Can you work these out from the model? Positions are in its coordinate system, mm. Round coordinates to 2 decimals unless told otherwise and drop trailing zeros. Loops run counter-clockwise (first coordinate to the right, second up) from the corner with the lowest first, then second, coordinate; pieces in that order, holes last. Notation, with made-up numbers: M -17.75,33 L 1.25,33 A20 cw 1.25,58 Z; hole C 2,80.5 d3. An arc over 180 degrees is marked long. Use a Markdown table: item, result. Add a question column.
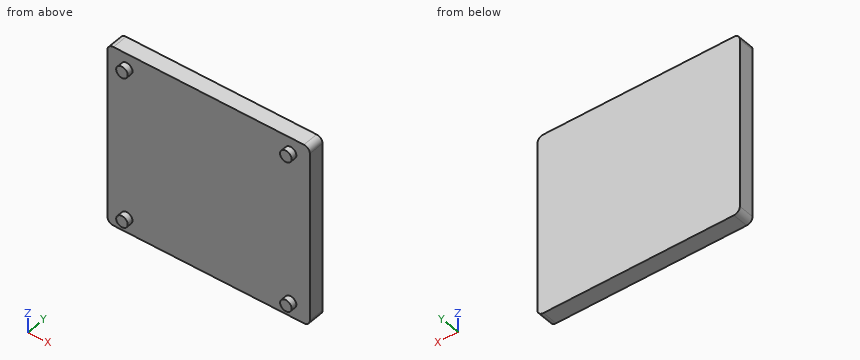
```python
from build123d import *

# Parameters (mm, degrees)
F0_R     = 1.45
F1_DEPTH = 4
F2_DEPTH = 5.5


with BuildPart() as f1:
    # F0 (on Front) → F1 (new body)
    with BuildSketch(Plane.XZ):
        with BuildLine():
            Line((23.95, 22.9), (-23.95, 22.9))
            ThreePointArc((-23.95, 22.9), (-25.01066, 22.46066), (-25.45, 21.4))
            Line((-25.45, 21.4), (-25.45, -21.4))
            ThreePointArc((-25.45, -21.4), (-25.01066, -22.46066), (-23.95, -22.9))
            Line((-23.95, -22.9), (23.95, -22.9))
            ThreePointArc((23.95, -22.9), (25.01066, -22.46066), (25.45, -21.4))
            Line((25.45, -21.4), (25.45, 21.4))
            ThreePointArc((25.45, 21.4), (25.01066, 22.46066), (23.95, 22.9))
        make_face()
        with Locations((-20.6, -19.15)):
            Circle(F0_R, mode=Mode.SUBTRACT)
        with Locations((20.6, -19.15)):
            Circle(F0_R, mode=Mode.SUBTRACT)
        with Locations((-20.6, 19.15)):
            Circle(F0_R, mode=Mode.SUBTRACT)
        with Locations((20.6, 19.15)):
            Circle(F0_R, mode=Mode.SUBTRACT)
        with Locations((20.6, 19.15)):
            Circle(F0_R)
        with Locations((-20.6, 19.15)):
            Circle(F0_R)
        with Locations((-20.6, -19.15)):
            Circle(F0_R)
        with Locations((20.6, -19.15)):
            Circle(F0_R)
    extrude(amount=F1_DEPTH)

    # F0 (on Front) → F2 (join)
    with BuildSketch(Plane.XZ):
        with Locations((-20.6, -19.15)):
            Circle(F0_R)
        with Locations((-20.6, 19.15)):
            Circle(F0_R)
        with Locations((20.6, 19.15)):
            Circle(F0_R)
        with Locations((20.6, -19.15)):
            Circle(F0_R)
    extrude(amount=F2_DEPTH)


solid = f1.part
```
(1) Suppose I cut it at B-B on z = 19.15. List the corners of the cut face in (x, y) for me.
(2) I'm going to push a flat-ended pin straight in: pin 1 (8 mm diameter, centred on x = 19.5, z = -13.5, fed in from -Y). Where does the tip first touch, or does it pass through?
(3) Suppose I cut it at C-C on x = -8.5. List the corners of the cut face in (y, z) for me.
(4) If I drill on probe 1 along Y at (x, z) = (8.5, -11.5); probe 2 along X at (y, z) = (-4.4, 19.5), over which ranges is the centre line in solid material (lowest first)? Write a range as [from, to].
(5) Suppose I cut it at A-A on x = -20.6. List the corners of the cut face in (y, z) for me, and give its area (3 significant figures).
(6) Suppose I cut it at D-D on z = -15.5. List the corners of the cut face in (x, y) for me, and give its area (3 significant figures).
Results below:
| question | item | result |
|---|---|---|
| 1 | outline | M -25.45,-4 L -22.05,-4 L -22.05,-5.5 L -19.15,-5.5 L -19.15,-4 L 19.15,-4 L 19.15,-5.5 L 22.05,-5.5 L 22.05,-4 L 25.45,-4 L 25.45,0 L -25.45,0 Z |
| 2 | pin 1 | stops at y = -4 |
| 3 | outline | M -4,-22.9 L 0,-22.9 L 0,22.9 L -4,22.9 Z |
| 4 | probe 1 | y = [-4, 0] |
| 4 | probe 2 | x = [-22.01, -19.19], [19.19, 22.01] |
| 5 | outline | M -5.5,-20.6 L -4,-20.6 L -4,-22.9 L 0,-22.9 L 0,22.9 L -4,22.9 L -4,20.6 L -5.5,20.6 L -5.5,17.7 L -4,17.7 L -4,-17.7 L -5.5,-17.7 Z |
| 5 | area | 192 mm² |
| 6 | outline | M -25.45,-4 L 25.45,-4 L 25.45,0 L -25.45,0 Z |
| 6 | area | 204 mm² |
